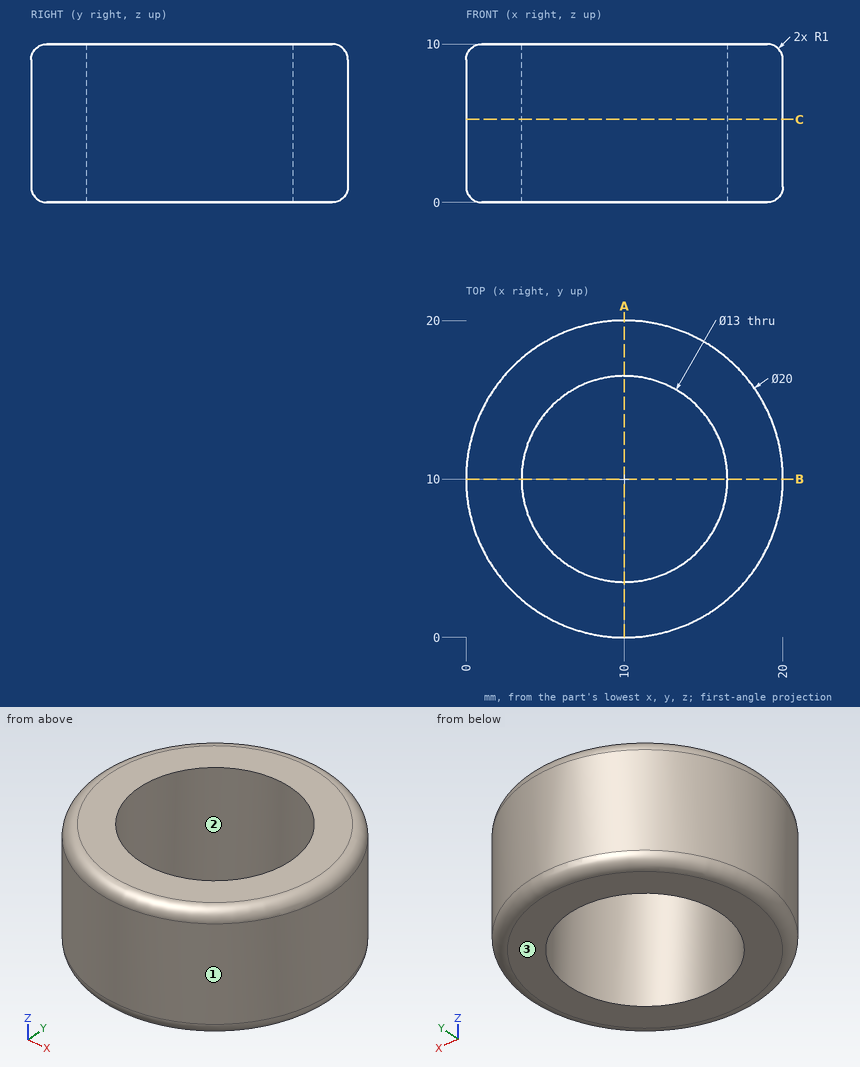
Study the drawing (mm; zero at the part's minimum x, y, z) and answer. Give positions to 0.01 mm unless a question says otherwise; leave off trailing zeros. Write each loop counter-clockwise with the first axis right and the second up, starting at its lowest first coordinate (ties: lowest second). Pieces come first, ordered by that corner, then holes.
(1) Flat-ended cylindrical pins translate along their axes: pin 1 Ø1 at (x, z) = (7, 1) entering from -Y; pin 2 Ø5 at (x, z) = (14, 5) entering from +Y. Find the tip coordinate at first contact, or state that the pin passes through.
Final values:
pin 1: stops at y = 0.32
pin 2: stops at y = 19.89
(2) Straight lines are drawn through the part: line 1 (Y direction, x = 10, z = 3.75); line 2 (Y direction, x = 8.5, z = 9); line 3 (X direction, y = 4, z = 4.5). For each, find the intervals that lie inside material, in ascending order.
Final values:
line 1: y = 0 to 3.5, 16.5 to 20
line 2: y = 0.11 to 3.68, 16.32 to 19.89
line 3: x = 2 to 7.5, 12.5 to 18
(3) The part is cut by section A-A on x = 10. Write down the section's boundary in (y, z).
Final values:
outline: (0, 1) arc R1 ccw to (1, 0) - (3.5, 0) - (3.5, 10) - (1, 10) arc R1 ccw to (0, 9) - close; (16.5, 0) - (19, 0) arc R1 ccw to (20, 1) - (20, 9) arc R1 ccw to (19, 10) - (16.5, 10) - close
(4) The part is cut by section C-C on z = 5.25. Write down the section's boundary in (x, y).
Final values:
outline: circle Ø20 at (10, 10); hole circle Ø13 at (10, 10)
(5) The mould has two halves that part along X. Classify the marked faces 1, 2 and 3: pulls with the +X half, pulls with the -X half, needs draft (parallel to the pull), parting line crosses it, or undercut.
Final values:
face 1: parting line crosses it
face 2: undercut
face 3: needs draft
